from build123d import *

# Parameters (mm, degrees)
SKETCH_1_R      = 2
SKETCH_1_R_2    = 2.08
SKETCH_1_R_3    = 5
EXTRUDE_2_DEPTH = 2


with BuildPart() as part:
    # 草图1 → 凸台-拉伸2 (new body)
    with BuildSketch(Plane.XY):
        with BuildLine():
            Line((-41, -12.75), (-37, -12.75))
            Line((-37, -12.75), (-37, -15.75))
            Line((-37, -15.75), (-30, -15.75))
            Line((-30, -15.75), (-30, -12.75))
            Line((-30, -12.75), (-25.488968202, -12.75))
            ThreePointArc((-25.488968202, -12.75), (0, -28.5), (25.488968202, -12.75))
            Line((25.488968202, -12.75), (30, -12.75))
            Line((30, -12.75), (30, -15.75))
            Line((30, -15.75), (37, -15.75))
            Line((37, -15.75), (37, -12.75))
            Line((37, -12.75), (41, -12.75))
            Line((41, -12.75), (41, -9.5))
            Line((41, -9.5), (44, -9.5))
            Line((44, -9.5), (44, -4.5))
            Line((44, -4.5), (41, -4.5))
            Line((41, -4.5), (41, 4.5))
            Line((41, 4.5), (44, 4.5))
            Line((44, 4.5), (44, 9.5))
            Line((44, 9.5), (41, 9.5))
            Line((41, 9.5), (41, 12.75))
            Line((41, 12.75), (37, 12.75))
            Line((37, 12.75), (37, 15.75))
            Line((37, 15.75), (30, 15.75))
            Line((30, 15.75), (30, 12.75))
            Line((30, 12.75), (25.488968202, 12.75))
            ThreePointArc((25.488968202, 12.75), (0, 28.5), (-25.488968202, 12.75))
            Line((-25.488968202, 12.75), (-30, 12.75))
            Line((-30, 12.75), (-30, 15.75))
            Line((-30, 15.75), (-37, 15.75))
            Line((-37, 15.75), (-37, 12.75))
            Line((-37, 12.75), (-41, 12.75))
            Line((-41, 12.75), (-41, 9.5))
            Line((-41, 9.5), (-44, 9.5))
            Line((-44, 9.5), (-44, 4.5))
            Line((-44, 4.5), (-41, 4.5))
            Line((-41, 4.5), (-41, -4.5))
            Line((-41, -4.5), (-44, -4.5))
            Line((-44, -4.5), (-44, -9.5))
            Line((-44, -9.5), (-41, -9.5))
            Line((-41, -9.5), (-41, -12.75))
        make_face()
        with Locations((12.990381057, 7.5)):
            Circle(SKETCH_1_R, mode=Mode.SUBTRACT)
        with Locations((0, 14.25)):
            Circle(SKETCH_1_R_2, mode=Mode.SUBTRACT)
        with Locations((-12.990381057, 7.5)):
            Circle(SKETCH_1_R, mode=Mode.SUBTRACT)
        with Locations((-12.340862004, -7.125)):
            Circle(SKETCH_1_R_2, mode=Mode.SUBTRACT)
        with Locations((0, -15)):
            Circle(SKETCH_1_R, mode=Mode.SUBTRACT)
        with Locations((12.340862004, -7.125)):
            Circle(SKETCH_1_R_2, mode=Mode.SUBTRACT)
        Circle(SKETCH_1_R_3, mode=Mode.SUBTRACT)
    extrude(amount=EXTRUDE_2_DEPTH)


solid = part.part
The listing builds one solid part. Answer for the finished solid, in the listing's coordinates (mm). A direction names the side the tool comes from. Give positions to 0.01 mm unless a question says otherwise; leave off trailing zeros. Order: outer loops, then holes, each group sorted by start corner. A loop starts at its lowest first (then second) coordinate and runs counter-clockwise, first axis right, second up. Notation, with made-up numbers: (28.25, 8) - (43.25, 8) arc R31 ccw to (43.25, 41) - close; hole circle Ø6 at (-37.5, -19). An arc over 180 degrees is marked (long way). Answer as CSV lines item,"result".
Q1. A cutting plane is placed at A-A, the plane x = 0. Determine the outline of the cut face in (y, z).
Answer key:
outline,"(-28.5, 0) - (-17, 0) - (-17, 2) - (-28.5, 2) - close; (-13, 0) - (-5, 0) - (-5, 2) - (-13, 2) - close; (5, 0) - (12.17, 0) - (12.17, 2) - (5, 2) - close; (16.33, 0) - (28.5, 0) - (28.5, 2) - (16.33, 2) - close"
Q2. A cutting plane is placed at C-C, the plane y = -3. Determine the outline of the cut face in (x, z).
Answer key:
outline,"(-41, 0) - (-4, 0) - (-4, 2) - (-41, 2) - close; (4, 0) - (41, 0) - (41, 2) - (4, 2) - close"
Q3. Each of these flat-tipped pins is pushed along its axis until it touches: pin 1 Ø0.6 at (x, z) = (-33, 1) entering from +Y; pin 2 Ø0.6 at (x, z) = (27, 1) entering from +Y; pin 3 Ø0.6 at (x, z) = (-28.5, 1) entering from -Y. Where does it stop, or does it pass through?
Answer key:
pin 1,"stops at y = 15.75"
pin 2,"stops at y = 12.75"
pin 3,"stops at y = -12.75"
Q4. A cutting plane is placed at D-D, the plane y = 14.25. Determine the outline of the cut face in (x, z).
Answer key:
outline,"(-37, 0) - (-30, 0) - (-30, 2) - (-37, 2) - close; (-24.68, 0) - (-2.08, 0) - (-2.08, 2) - (-24.68, 2) - close; (2.08, 0) - (24.68, 0) - (24.68, 2) - (2.08, 2) - close; (30, 0) - (37, 0) - (37, 2) - (30, 2) - close"
Q5. Straight lines are drawn through the part: L1, parallel to Y at x = 11.5, z = 1.4; L2, parallel to Y at x = -0.5, z = 0.85; L3, parallel to Y at x = -1.5, z = 1.9. For each, find the intervals that lie inside material, in ascending order.
Answer key:
L1,"y = -26.08 to -9.03, -5.22 to 6.17, 8.83 to 26.08"
L2,"y = -28.5 to -16.94, -13.06 to -4.97, 4.97 to 12.23, 16.27 to 28.5"
L3,"y = -28.46 to -16.32, -13.68 to -4.77, 4.77 to 12.81, 15.69 to 28.46"
Q6. Which of the six approach directions +Z, -Z, +X, -X, +Y, -Y give full straight-line access (tool end or side, diameter ignored) to faces 1 (the face through (-34, -15.75, 1)), 2 (the face through (42, -9.5, 1)), 3 (the face through (30, 14, 1))?
Answer key:
face 1,"+Z, -Z, -X, -Y"
face 2,"+Z, -Z, +X, -Y"
face 3,"+Z, -Z, +Y"
Q7. A cutting plane is placed at B-B, the plane y = 7.5. Determine the outline of the cut face in (x, z).
Answer key:
outline,"(-44, 0) - (-14.99, 0) - (-14.99, 2) - (-44, 2) - close; (-10.99, 0) - (10.99, 0) - (10.99, 2) - (-10.99, 2) - close; (14.99, 0) - (44, 0) - (44, 2) - (14.99, 2) - close"
Q8. Determine the mould class of faces 4 (the face through (28, -12.75, 1)), 5 (the face through (43, 9.5, 1)), 6 (the face through (-30, -14, 1)), 7 (the face through (41, 11, 1)) for opening direction X: pulls with the +X half, pulls with the -X half, needs draft (parallel to the pull), parting line crosses it, or undercut.
Answer key:
face 4,"undercut"
face 5,"needs draft"
face 6,"undercut"
face 7,"pulls with the +X half"
